from build123d import *

# Parameters (mm, degrees)
F2_DEPTH = 60
F3_DEPTH = 52
F4_W     = 10.2412812412
F4_H     = 20.4825601541
F4_W_2   = 10.6680002064
F4_H_2   = 20.9092802834
F4_W_3   = 10.0279208273
F4_H_3   = 21.9760797918
F4_W_4   = 10.8813615516
F4_H_4   = 22.402798757
F5_DEPTH = 29.8242783788
F6_W     = 10.4546393268
F6_H     = 20.9092812147
F7_DEPTH = 29.8242783788


# Not quite as in the source:
# - ends of sketch curves that miss each other by under 0.0002 mm in the source are joined


with BuildPart() as f2:
    # F0 (on Top) → F2 (new body)
    with BuildSketch(Plane.XY):
        Polygon((-14.9116391894, 32.3240421712), (-14.9116391894, 24.8527319824), (-14.9116391894, -24.8527319824), (-14.9116391894, -32.3240421712), (14.9116391894, -32.3240421712), (14.9116391894, -24.8527319824), (14.9116391894, 24.8527319824), (14.9116391894, 32.3240421712), align=None)
        Polygon((-7.4186391894, 24.8527319824), (-0.0743608106, 24.8527319824), (0.0743608106, 24.8527319824), (7.4186391894, 24.8527319824), (7.4186391894, 0), (7.4186391894, -24.8527319824), (-7.4186391894, -24.8527319824), (-7.4186391894, 0), align=None, mode=Mode.SUBTRACT)
        Polygon((0.0743608106, 24.8527319824), (-0.0743608106, 24.8527319824), (-7.4186391894, 24.8527319824), (-7.4186391894, 0), (-7.4186391894, -24.8527319824), (7.4186391894, -24.8527319824), (7.4186391894, 0), (7.4186391894, 24.8527319824), align=None)
    extrude(amount=-F2_DEPTH)

    # F1 (on face) → F3 (cut)
    with BuildSketch(Plane.XY):
        Polygon((7.4186391894, 24.8527319824), (0.0743608106, 24.8527319824), (-0.0743608106, 24.8527319824), (-7.4186391894, 24.8527319824), (-7.4186391894, 0), (-7.4186391894, -24.8527319824), (7.4186391894, -24.8527319824), (7.4186391894, 0), align=None)
    extrude(amount=-F3_DEPTH, mode=Mode.SUBTRACT)

    # F4 (on face) → F5 (cut, through all)
    with BuildSketch(Plane.YZ.offset(14.9116391894)):
        with Locations((-22.8295195848, -14.401800232)):
            Rectangle(F4_W, F4_H)
        with Locations((-7.2542401031, -14.1884401673)):
            Rectangle(F4_W_2, F4_H_2)
        with Locations((7.2542401031, -14.1884401673)):
            Rectangle(F4_W_2, F4_H_2)
        with Locations((22.8295195848, -14.401800232)):
            Rectangle(F4_W, F4_H)
        with Locations((22.7228393778, -40.3250399977)):
            Rectangle(F4_W_3, F4_H_3)
        with Locations((7.5742793269, -40.1116805151)):
            Rectangle(F4_W_4, F4_H_4)
        with Locations((-7.5742793269, -40.1116805151)):
            Rectangle(F4_W_4, F4_H_4)
        with Locations((-22.7228393778, -40.3250399977)):
            Rectangle(F4_W_3, F4_H_3)
    extrude(amount=-F5_DEPTH, mode=Mode.SUBTRACT)

    # F6 (on face) → F7 (cut, through all)
    with BuildSketch(Plane(origin=(-14.9116391894, 0, 0), x_dir=(0, -1, 0), z_dir=(-1, 0, 0))):
        Polygon((12.5882383436, 0), (-12.3748793267, 0), (-12.3748793267, -3.7338000257), (-1.9202399999, -3.7338000257), (-1.9202399999, -24.643080309), (1.9202399999, -24.6430812404), (1.9202399999, -3.7338000257), (12.5882402062, -3.7338000257), align=None)
        with Locations((-7.1475596633, -14.188440633)):
            Rectangle(F6_W, F6_H)
        Polygon((12.5882383436, -24.6430812404), (12.5882383436, -3.7338000257), (1.9202399999, -3.7338000257), (1.9202399999, -24.643080309), align=None)
    extrude(amount=-F7_DEPTH, mode=Mode.SUBTRACT)


solid = f2.part
Geometry: final body of the model. Coordinates: model frame, mm. A direction names the side the tool comes from. Give positions to 0.01 mm unless a question says otherwise; leave off trailing zeros. Loops run counter-clockwise (first coordinate to the right, second up) from the corner with the lowest first, then second, coordinate; pieces in that order, holes last. Notation, with made-up numbers: (9, -26) - (61, -26) arc R29 ccw to (61, 10) - close; hole circle Ø7 at (14.5, 53.5). An arc over 180 degrees is marked (long way). Answer as CSV lines item,"result". Start each with the question number.
1. Draft query along X for faces 4 (the face through (0, -24.853, -2)), 5 (the face through (14.912, 0, -30)), 6 (the face through (11, 12.588, -14)). Return one class per face: released by +X, released by -X, zero draft, split by the parting line, or undercut.
2. Pin query (flat end, axial travel): P1, Ø5, axis at x = 2.5, y = -17, coming from the +Z side; P2, Ø4, axis at x = 10.5, y = 0.5, coming from the +Z side. Return the tip coordinate at first contact, or that it passes through.
3. Section D-D, the plane z = -50. Give the number of separate pieces and of enclosed holes in the cut face, plus the area to 3 significant figures.
4. Reachability of faces 1 (the face through (7.419, 0, -26)), 2 (the face through (-11, 7, -24.643)), 3 (the face through (0.2, -25.2, -24.643)) from +Z, -Z, +X, -X, +Y, -Y: full face, straight path, thin tool, end or side. Return the list, or none.
5. Ray query, L1, parallel to Y at x = -12, z = -13; L2, parallel to Y at x = -9.75, z = -33.5; L3, parallel to Y at x = 7, z = -14.5. Return the intervals inside material, ascending.
6. Section A-A, the plane y = 23.5. Return loops of the section in (x, z).
7. Section C-C, the plane z = -12. Return loops of the section in (x, y), plus the area to 3 significant figures.
8. Section B-B, the plane y = -5. Return loops of the section in (x, z).
Answers:
1,face 4,"undercut"
1,face 5,"released by +X"
1,face 6,"zero draft"
2,P1,"stops at z = -52"
2,P2,"stops at z = -24.64"
3,separate pieces,"8"
3,enclosed holes,"0"
3,area,"478 mm2"
4,face 1,"+Z"
4,face 2,"+Z, +X, -X"
4,face 3,"+X, -X"
5,L1,"y = -32.32 to -27.95, -17.71 to -12.59, 12.59 to 17.71, 27.95 to 32.32"
5,L2,"y = -32.32 to -27.74, -17.71 to -13.01, -2.13 to 2.13, 13.01 to 17.71, 27.74 to 32.32"
5,L3,"y = -32.32 to -27.95, 27.95 to 32.32"
6,outline,"(-14.91, -60) - (14.91, -60) - (14.91, -51.31) - (7.42, -51.31) - (7.42, -52) - (-7.42, -52) - (-7.42, -51.31) - (-14.91, -51.31) - close; (-14.91, -29.34) - (-7.42, -29.34) - (-7.42, -24.64) - (-14.91, -24.64) - close; (-14.91, -4.16) - (-7.42, -4.16) - (-7.42, 0) - (-14.91, 0) - close; (7.42, -29.34) - (14.91, -29.34) - (14.91, -24.64) - (7.42, -24.64) - close; (7.42, -4.16) - (14.91, -4.16) - (14.91, 0) - (7.42, 0) - close"
7,outline,"(-14.91, -32.32) - (14.91, -32.32) - (14.91, -27.95) - (-14.91, -27.95) - close; (-14.91, -17.71) - (-7.42, -17.71) - (-7.42, -12.59) - (-14.91, -12.59) - close; (-14.91, 12.59) - (-7.42, 12.59) - (-7.42, 17.71) - (-14.91, 17.71) - close; (-14.91, 27.95) - (14.91, 27.95) - (14.91, 32.32) - (-14.91, 32.32) - close; (7.42, -17.71) - (14.91, -17.71) - (14.91, -12.59) - (7.42, -12.59) - close; (7.42, 12.59) - (14.91, 12.59) - (14.91, 17.71) - (7.42, 17.71) - close"
7,area,"414 mm2"
8,outline,"(-14.91, -60) - (14.91, -60) - (14.91, -51.31) - (7.42, -51.31) - (7.42, -52) - (-7.42, -52) - (-7.42, -51.31) - (-14.91, -51.31) - close; (-14.91, -28.91) - (-7.42, -28.91) - (-7.42, -24.64) - (-14.91, -24.64) - close; (7.42, -28.91) - (14.91, -28.91) - (14.91, -24.64) - (7.42, -24.64) - close"
